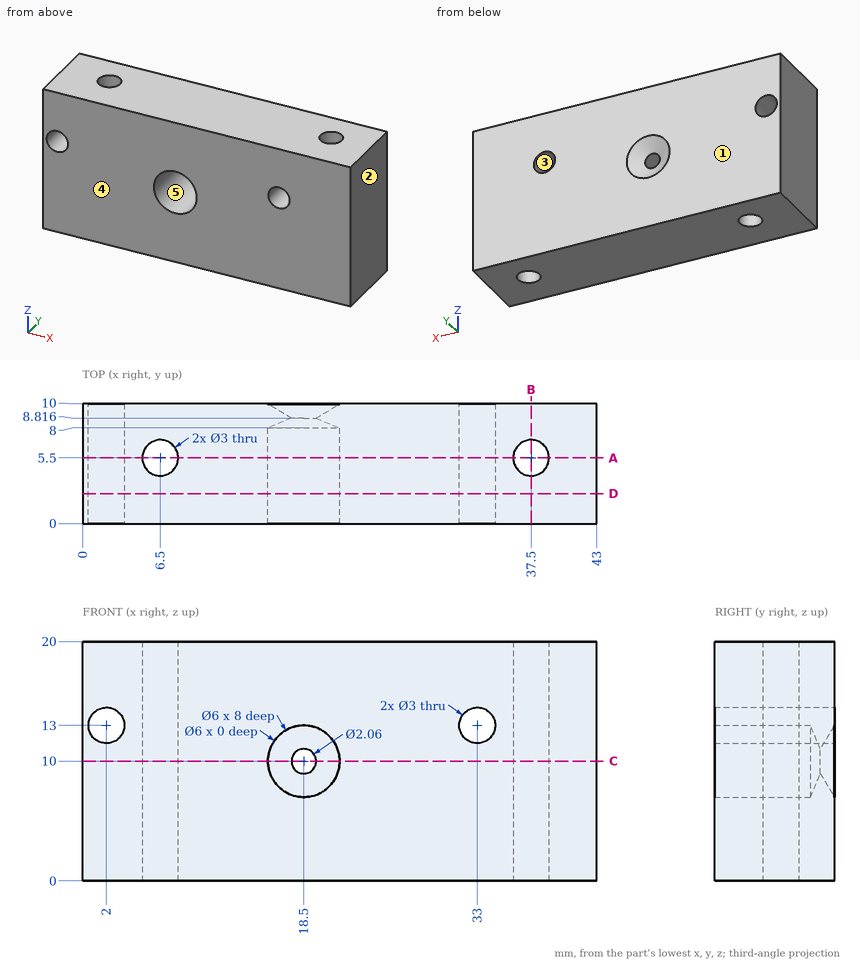
Here's the drawing with two shaded views (mm, measured from the low corner). I have some questions. A direction names the side the tool comes from. Coordinates: 2 decimals unless noted, no trailing zeros. Order: outer loops, then holes, each group sorted by start corner. A loop starts at its lowest first (then second) coordinate and runs counter-clockwise, first axis right, second up. Notation, with made-up numbers: (10, -24) - (66, -24) arc R36 cw to (66, 13) - close; hole circle Ø1 at (89.25, 12). An arc over 180 degrees is marked (long way). Answer in a Markdown table with one row per item.
1. Suppose I cut it at B-B (x = 37.5). Please give me the cut outline in (y, z), and give its area (3 significant figures).
Reply:
| item | result |
|---|---|
| outline | (0, 0) - (4, 0) - (4, 20) - (0, 20) - close; (7, 0) - (10, 0) - (10, 20) - (7, 20) - close |
| area | 140 mm^2 |
2. If we mould it in two halves opening along X, with no side actions, what happens to the marked faces 1, 2 and 3? For each: pulls with the +X half, pulls with the -X half, needs draft (parallel to the pull), parting line crosses it, or undercut.
Reply:
| item | result |
|---|---|
| face 1 | needs draft |
| face 2 | pulls with the +X half |
| face 3 | undercut |
3. Suppose I cut it at C-C (z = 10). Give the number of separate pieces and of enclosed holes in the cut face, and give its area (3 significant figures).
Reply:
| item | result |
|---|---|
| separate pieces | 2 |
| enclosed holes | 2 |
| area | 360 mm^2 |
4. For pin 1 (5.5 mm diameter, centred on x = 18.5, z = 10, fed in from +Y); pin 2 (1 mm diameter, centred on x = 19, z = 7.5, fed in from -Y); pin 3 (5.5 mm diameter, centred on x = 18.5, z = 10, fed in from -Y), each with a flat end and sliding along its axis, tell me the tip position at first contact or that it passes through.
Reply:
| item | result |
|---|---|
| pin 1 | stops at y = 9.85 |
| pin 2 | stops at y = 0 |
| pin 3 | stops at y = 8.1 |
5. Suppose I cut it at D-D (y = 2.5). Please give me the cut outline in (x, z).
Reply:
| item | result |
|---|---|
| outline | (0, 0) - (43, 0) - (43, 20) - (0, 20) - close; hole circle Ø3 at (2, 13); hole circle Ø6 at (18.5, 10); hole circle Ø3 at (33, 13) |
6. If I drill on line 1 along X through (y, z) = (2, 10); line 2 along Z through (x, y) = (33, 8.5); line 3 along X through (y, z) = (4.5, 10), over which ranges is the centre line in solid material (lowest first)?
Reply:
| item | result |
|---|---|
| line 1 | x = 0 to 15.5, 21.5 to 43 |
| line 2 | z = 0 to 11.5, 14.5 to 20 |
| line 3 | x = 0 to 5.38, 7.62 to 15.5, 21.5 to 36.38, 38.62 to 43 |
7. For the marked faces 4 and 5, which set-ups out of +Z, -Z, +X, -X, +Y, -Y let a thin tool reach every point of the face, with its end or its side?
Reply:
| item | result |
|---|---|
| face 4 | +Z, -Z, +X, -X, -Y |
| face 5 | -Y |
8. Suppose I cut it at A-A (y = 5.5). Please give me the cut outline in (x, z).
Reply:
| item | result |
|---|---|
| outline | (0, 0) - (5, 0) - (5, 20) - (0, 20) - close; (8, 0) - (36, 0) - (36, 20) - (8, 20) - close; (39, 0) - (43, 0) - (43, 20) - (39, 20) - close; hole circle Ø3 at (2, 13); hole circle Ø6 at (18.5, 10); hole circle Ø3 at (33, 13) |
